Autodesk Inventor part; units mm, degrees
ref_plane "Work Plane4" through (-24.55, -10, -34.5672) normal (0, -1, 0) x (1, 0, 0)
ref_plane "Work Plane5" through (-19.3, -32.4, 0) normal (0, 0, 1) x (1, 0, 0)
ref_plane "YZ Plane" through (0, 0, 0) normal (1, 0, 0) x (0, 1, 0)
ref_plane "Work Plane1" through (26.5, 0, 0) normal (0, 0, -1) x (-1, 0, 0)
sketch "Sketch1" plane through (-19.3, 0, 0) normal (0, 0, 1) x (1, 0, 0)
  circle A0 centre (2.9, -26.2) radius 1.75
  circle A1 centre (2.9, -6.2) radius 1.75
  circle A2 centre (22.9, -26.2) radius 1.75
  circle A3 centre (22.9, -6.2) radius 1.75
  line L0 (0.3744, -33.9) -> (0.3744, 2.1) construction
  line L1 (25.8, 0) -> (25.8, -32.4) construction
  line L2 (-0.6, 0) -> (-0.6, -32.4) construction
  line L3 (19.3, -32.4) -> (25.8, -32.4) construction
  line L4 (25.8, 0) -> (25.8, -32.4) construction
  line L5 (19.3, 0) -> (25.8, 0) construction
  line L6 (19.3, 0) -> (19.3, -32.4) construction
  circle A4 centre (22.9, -6.2) radius 1.75 construction
  circle A5 centre (22.9, -26.2) radius 1.75 construction
  line L7 (0, -32.4) -> (6.5, -32.4) construction
  line L8 (6.5, 0) -> (6.5, -32.4) construction
  line L9 (0, 0) -> (6.5, 0) construction
  line L10 (0, 0) -> (0, -32.4) construction
  circle A6 centre (2.9, -6.2) radius 1.75 construction
  circle A7 centre (2.9, -26.2) radius 1.75 construction
  line L11 (29.4, -10) -> (-3.6, -10)
  line L12 (-3.6, -10) -> (-3.6, 0)
  line L13 (-3.6, 0) -> (29.4, 0)
  line L14 (29.4, 0) -> (29.4, -10)
  circle A8 centre (22.9, -26.2) radius 2.25
  circle A9 centre (22.9, -6.2) radius 2.25
  circle A10 centre (2.9, -6.2) radius 2.25
  circle A11 centre (2.9, -26.2) radius 2.25
  line L15 (26.4, 0) -> (26.4, -32.4)
  dimension "d1" = 3
  dimension "d2" = 0.5
  dimension "d3" = 0.5
  dimension "d4" = 0.5
  dimension "d5" = 0.5
  dimension "d19" = 3
  dimension "d32" = 10
extrude "Extrusion1" add sketch "Sketch1" along normal blind 5 contours L11 L15 L13 L14 | L11 L12 L13 L15
sketch "Sketch2" plane through (-19.3, 0, 0) normal (0, 0, -1) x (-1, 0, 0)
  circle A0 centre (-2.9, -6.2) radius 2.25
  circle A1 centre (-22.9, -6.2) radius 2.25
  line L0 (3.6, -10) -> (-29.4, -10)
  line L1 (-29.4, -10) -> (-29.4, 0)
  line L2 (-29.4, 0) -> (3.6, 0)
  line L3 (3.6, 0) -> (3.6, -10)
  line L4 (3.6, -10) -> (3.6, 0)
  line L5 (3.6, 0) -> (0.8, 0)
  line L6 (0.8, 0) -> (0.8, -10)
  line L7 (0.8, -10) -> (3.6, -10)
  line L8 (3.6, -10) -> (3.6, 0)
  line L9 (-29.4, -10) -> (3.6, -10)
  line L10 (-29.4, 0) -> (-26.6, 0)
  line L11 (-26.6, 0) -> (-26.6, -10)
  line L12 (-26.6, -10) -> (-29.4, -10)
  line L13 (-29.4, -10) -> (-29.4, 0)
  point P0 (-19.3, 0)
  dimension "d8" = 2.8
  dimension "d9" = 2.8
  dimension "d10" = 0
extrude "Extrusion2" add sketch "Sketch2" along normal blind 12 contours L0 L6 L2 L3 | L0 L1 L2 L11
sketch "Sketch3" plane through (-19.3, 0, -12) normal (0, 0, -1) x (-1, 0, 0)
  line L0 (-29.4, 0) -> (-29.4, -10)
  line L1 (-29.4, -10) -> (-26.6, -10)
  line L2 (-26.6, -10) -> (-26.6, 0)
  line L3 (-26.6, 0) -> (-29.4, 0)
  line L4 (3.6, -10) -> (3.6, 0)
  line L5 (3.6, 0) -> (0.8, 0)
  line L6 (0.8, 0) -> (0.8, -10)
  line L7 (-18.8691, 0.2794) -> (-18.8691, -79.7206) construction
  line L8 (-8.1725, 0.2794) -> (-8.1725, -79.7206) construction
  line L9 (-29.4, 0) -> (3.6, 0) construction
  line L10 (3.6, -10) -> (-29.4, -10)
  line L11 (-29.4, 0) -> (-20.4, 0)
  line L12 (-20.4, 0) -> (-20.4, -10)
  line L13 (-20.4, -10) -> (-29.4, -10)
  line L14 (-29.4, -10) -> (-29.4, 0)
  line L15 (3.6, 0) -> (3.6, -10)
  line L16 (3.6, 0) -> (-5.4, 0)
  line L17 (-5.4, 0) -> (-5.4, -10)
  line L18 (-5.4, -10) -> (3.6, -10)
  line L19 (3.6, -10) -> (3.6, 0)
  line L20 (0.8, -10) -> (3.6, -10)
  point P0 (-19.3, 0)
  dimension "d13" = 9
  dimension "d14" = 9
extrude "Extrusion3" add sketch "Sketch3" along normal blind 1 and the other way blind 1
ref_plane "Work Plane2" through (-22.9, -4, 5) normal (0, 1, 0) x (1, 0, 0)
sketch "Sketch4" plane through (-22.9, -10, 5) normal (0, 1, 0) x (1, 0, 0)
  line L0 (0, 0) -> (0, 18)
  line L1 (33, 0) -> (0, 0)
  line L2 (33, 0) -> (33, 18)
  line L3 (24, 18) -> (33, 18)
  line L4 (24, 18) -> (24, 16)
  line L5 (30.2, 16) -> (24, 16)
  line L6 (30.2, 5) -> (30.2, 16)
  line L7 (2.8, 5) -> (30.2, 5)
  line L8 (2.8, 5) -> (2.8, 16)
  line L9 (9, 16) -> (2.8, 16)
  line L10 (9, 16) -> (9, 18)
  line L11 (0, 18) -> (9, 18)
  line L12 (32.9002, 18.2) -> (30.3433, 20.7569) construction
  line L13 (-0.4956, 21.98) -> (-4.2756, 18.2) construction
  line L14 (34.2709, 21.1536) -> (36.398, 19.0265) construction
  line L15 (30.3433, 26.08) -> (30.3433, 18.1) construction
  line L16 (21.9706, 26.08) -> (21.9706, 18.1) construction
  line L17 (11.0029, 26.08) -> (11.0029, 18.1) construction
  line L18 (2.6055, 26.08) -> (2.6055, 20.7569) construction
  line L19 (24, 18) -> (33, 18)
  line L20 (31.5357, 18) -> (29.8433, 19.6923)
  line L21 (29.8433, 19.6923) -> (22.4706, 19.6923)
  line L22 (22.4706, 19.6923) -> (24, 16)
  line L23 (29.8433, 19.6923) -> (29.8433, 37.6831)
  line L24 (22.4706, 19.6923) -> (29.8433, 19.6923)
  line L25 (29.8433, 19.6923) -> (29.8433, 37.6831)
  line L26 (29.8433, 37.6831) -> (22.4706, 37.6831)
  line L27 (22.4706, 37.6831) -> (22.4706, 19.6923)
  point P0 (22.9, 5)
  dimension "d21" = 157.5
  dimension "d22" = 0.5
  dimension "d23" = 0.5
extrude "Extrusion4" add sketch "Sketch4" along normal blind 5
ref_plane "Work Plane3" through (-6.4, -10, 5) normal (-1, 0, 0) x (0, 0, 1)
mirror "Mirror1" about plane through (-6.4, -10, 5) normal (-1, 0, 0) of "Extrusion4"
chamfer "Chamfer2" distance 1 angle 45 4 edges at (9.3678, -10, -13) (-22.1678, -10, -13) (-17.6678, -5, -13) (4.8678, -5, -13)
sketch "Sketch5" plane through (-22.9, -5, 5) normal (0, 1, 0) x (1, 0, 0)
  line L0 (24, 19) -> (24, 16)
  line L1 (30.5357, 19) -> (24, 19)
  line L2 (30.5357, 19) -> (29.8433, 19.6923)
  line L3 (29.8433, 19.6923) -> (29.8433, 37.6831)
  line L4 (29.8433, 37.6831) -> (22.4706, 37.6831)
  line L5 (22.4706, 37.6831) -> (22.4706, 19.6923)
  line L6 (22.4706, 19.6923) -> (24, 16)
  line L7 (9, 19) -> (2.4643, 19)
  line L8 (9, 16) -> (9, 19)
  line L9 (10.5294, 19.6923) -> (9, 16)
  line L10 (10.5294, 37.6831) -> (10.5294, 19.6923)
  line L11 (3.1567, 37.6831) -> (10.5294, 37.6831)
  line L12 (3.1567, 19.6923) -> (3.1567, 37.6831)
  line L13 (2.4643, 19) -> (3.1567, 19.6923)
  circle A0 centre (26.1569, 33.9967) radius 3.6864
  circle A1 centre (6.843, 33.9967) radius 3.6864
  circle A2 centre (26.1569, 33.9967) radius 1.4
  circle A3 centre (6.843, 33.9967) radius 1.4
  circle A4 centre (26.1569, 28.9967) radius 1.4
  circle A5 centre (6.843, 28.9967) radius 1.4
  point P0 (22.9, 5)
  dimension "d33" = 2.8
  dimension "d34" = 2.8
  dimension "d37" = 2.8
  dimension "d38" = 2.8
  dimension "d39" = 5
  dimension "d40" = 5
extrude "Extrusion5" cut sketch "Sketch5" against normal through all contours A4 A0 | A0 A4 | A5 A1 | A1 A5 | A2 | A3 picked at (26.2031, 30.3641) picked at (26.0901, 28.5093) picked at (6.8892, 30.3641) picked at (6.7762, 28.5093)
sketch "Sketch6" plane through (-22.9, -10, 5) normal (0, 1, 0) x (1, 0, 0)
  line L0 (0, 0) -> (0, 18)
  line L1 (33, 0) -> (0, 0)
  line L2 (33, 0) -> (33, 18)
  line L3 (24, 18) -> (33, 18)
  line L4 (24, 18) -> (24, 16)
  line L5 (30.2, 16) -> (24, 16)
  line L6 (30.2, 5) -> (30.2, 16)
  line L7 (2.8, 5) -> (30.2, 5)
  line L8 (2.8, 5) -> (2.8, 16)
  line L9 (9, 16) -> (2.8, 16)
  line L10 (9, 16) -> (9, 18)
  line L11 (0, 18) -> (9, 18)
  circle A0 centre (15.4444, -9.8) radius 1.1933
  line L12 (0, 0) -> (11.4444, -13.8)
  line L13 (11.4444, -13.8) -> (19.4444, -13.8)
  line L14 (33, 0) -> (33, 18)
  line L15 (19.4444, -13.8) -> (33, 0)
  circle A1 centre (15.4444, -9.8) radius 2
  point P0 (22.9, 5)
  dimension "d41" = 4
  dimension "d42" = 4
  dimension "d43" = 4
  dimension "d44" = 4
ref_plane "Work Plane4" through (-24.55, -10, -34.5672) normal (0, -1, 0) x (1, 0, 0)
extrude "Extrusion6" add sketch "Sketch6" along normal up to surface (10 mm away) contours L1 L15 L13 L12
ref_plane "Work Plane5" through (-19.3, -32.4, 0) normal (0, 0, 1) x (1, 0, 0)
sketch "Sketch7" plane through (-19.3, 0, 5) normal (0, 0, 1) x (1, 0, 0)
  circle A0 centre (2.9, -6.2) radius 1.5
  circle A1 centre (22.9, -6.2) radius 1.25
  circle A2 centre (2.9, -6.2) radius 2.25
  circle A3 centre (22.9, -6.2) radius 2.25
  point P0 (19.3, 0)
  dimension "d47" = 4.5
  dimension "d48" = 4.5
extrude "Extrusion7" cut sketch "Sketch7" against normal up to surface (5 mm away) contours A0 | A1 | A2 | A3
sketch "Sketch8" plane through (-11.4556, -10, 18.8) normal (0, 0, 1) x (1, 0, 0)
  line L0 (0, 0) -> (8, 0)
  line L1 (8, 0) -> (8, 10)
  line L2 (0, 0) -> (0, 10)
  line L3 (2.5, 13.1294) -> (2.5, 10.1294)
  line L4 (5.5, 13.1294) -> (5.5, 10.1294)
  line L5 (1, 5) -> (7, 5)
  line L6 (7, 5) -> (7, 2)
  line L7 (7, 2) -> (1, 2)
  line L8 (1, 2) -> (1, 5)
  line L9 (1, 5) -> (7, 2) construction
  line L10 (7, 5) -> (1, 2) construction
  line L11 (8, 10) -> (0, 10)
  point P0 (11.4556, 10)
  point P1 (4, 3.5)
  dimension "d51" = 6
  dimension "d52" = 3
extrude "Extrusion8" cut sketch "Sketch8" against normal blind 8 contours L5 L6 L7 L8
sketch "Sketch9" plane through (-19.3, 0, 5) normal (0, 0, 1) x (1, 0, 0)
  circle A0 centre (2.9, -6.2) radius 1.75
  circle A1 centre (22.9, -6.2) radius 1.75
  circle A2 centre (2.9, -6.2) radius 2.25
  circle A3 centre (22.9, -6.2) radius 2.25
  point P0 (19.3, 0)
extrude "Extrusion9" cut sketch "Sketch9" along normal through all contours A0 | A1 | A2 | A3
chamfer "Chamfer3" distance 1 angle 45 2 edges at (10.1, -4.5, -13) (-22.9, -4.5, -13)
sketch "Sketch10" plane through (-20.1, 0, 0) normal (0, 1, 0) x (1, 0, 0)
  circle A0 centre (1.1444, -3.3) radius 1.25
  circle A1 centre (24.1444, -3.3) radius 1.25
  circle A2 centre (1.1444, -3.3) radius 1.45
  circle A3 centre (24.1444, -3.3) radius 1.45
  point P0 (20.1, 0)
  dimension "d60" = 2.9
  dimension "d61" = 2.9
extrude "Extrusion10" cut sketch "Sketch10" against normal through all contours A0 | A1 | A2 | A3
properties part number "30_Cube_Z_Focus_Drylin_NEMA_slide"
Work out the finished part from the listing and answer in its coordinate system (mm). A direction names the side the tool comes from. Give positions to 0.01 mm unless a question says otherwise; leave off trailing zeros. Loops run counter-clockwise (first coordinate to the right, second up) from the corner with the lowest first, then second, coordinate; pieces in that order, holes last. Notation, with made-up numbers: (69, -26) -> (93, -26) arc R12 ccw to (93, -11) -> close; hole circle Ø10 at (4.25, -26). An arc over 180 degrees is marked (long way). Put each result on its own line as item: value. Start each with the question number.
Item 1: The part is cut by section B-B (x = -16.4). Give the vertices of the cut face in (y, z).
Item 2: The part is cut by section A-A (z = -3.5). Give the vertices of the cut face in (x, y), then the cut area to 3 significant figures.
Item 3: The mould has two halves that part along Z. Classify faces 1 (the face through (-16, -8, -32.683)), 2 (the face through (-5, -8, 15)), 3 (the face through (-15.411, -7.465, -27.755)), 4 (the face through (4, -5, -11)): released by +Z, released by -Z, zero draft, split by the parting line, or undercut.
Item 4: The part is cut by section C-C (z = 3.3). Give the vertices of the cut face in (x, y).
Item 5: Find the intervals of material crossed by L1, parallel to X at y = -8.75, z = -6.5; L2, parallel to X at y = -7, z = -20.5; L3, parallel to X at y = -6.2, z = 5.5, in increasing order. Write a range as [from, to].
Item 6: Which of the six approach directions +Z, -Z, +X, -X, +Y, -Y give full straight-line access (tool end or side, diameter ignored) to faces 5 (the face through (6.943, -8, -24)), 6 (the face through (9.4, -9.5, -12.5)), 7 (the face through (-9.5, -5, 14))?
Item 7: The part is cut by section D-D (x = 3.6). State how many separate pieces and enclosed holes the cut face has, then the cut area to 3 significant figures.
Item 8: Each of these flat-tipped pins is pushed along its axis until it touches: P1, Ø1.9, axis at x = 5, y = -3.5, coming from the +Z side; P2, Ø4, axis at y = -2, z = 9, coming from the -X side; P3, Ø1, axis at x = -15, y = -3, coming from the +Z side. Where does it stop, or does it pass through?
Answers below:
1. outline: (-10, -32.68) -> (-5, -32.68) -> (-5, -30.35) -> (-10, -30.35) -> close; (-10, -27.64) -> (-5, -27.64) -> (-5, -25.35) -> (-10, -25.35) -> close; (-10, -22.64) -> (-5, -22.64) -> (-5, -14) -> (-4, -13) -> (0, -13) -> (0, -11) -> (-10, -11) -> close; (-10, 0) -> (-8.45, 0) -> (-8.45, 12.84) -> (-10, 12.84) -> close; (-3.95, 0) -> (0, 0) -> (0, 12.84) -> (-3.95, 12.84) -> close
2. outline: (-22.9, -10) -> (-20.1, -10) -> (-20.1, 0) -> (-22.9, 0) -> close; (7.3, -10) -> (10.1, -10) -> (10.1, 0) -> (7.3, 0) -> close
2. area: 56.0 mm2
3. face 1: released by -Z
3. face 2: zero draft
3. face 3: undercut
3. face 4: undercut
4. outline: (-22.9, -10) -> (-20.41, -10) -> (-20.41, 0) -> (-22.9, 0) -> close; (-17.51, -10) -> (2.59, -10) -> (2.59, -8.21) arc R2.25 cw to (2.59, -4.19) -> (2.59, 0) -> (-17.51, 0) -> (-17.51, -4.24) arc R2.25 cw (long way) to (-17.51, -8.16) -> close; (5.49, -10) -> (10.1, -10) -> (10.1, 0) -> (5.49, 0) -> (5.49, -4.99) arc R2.25 cw to (5.49, -7.41) -> close
5. L1: [-22.9, -20.1], [7.3, 10.1]
5. L2: [-19.74, -12.37], [-0.43, 6.94]
5. L3: [-22.49, -18.65], [-14.15, 1.35], [5.85, 9.61]
6. face 5: -Z, +X, +Y, -Y
6. face 6: -Z, +X, -Y
6. face 7: +Z
7. separate pieces: 7
7. enclosed holes: 0
7. area: 140 mm2
8. P1: z = 11.16
8. P2: x = -21.24
8. P3: z = 15.13
